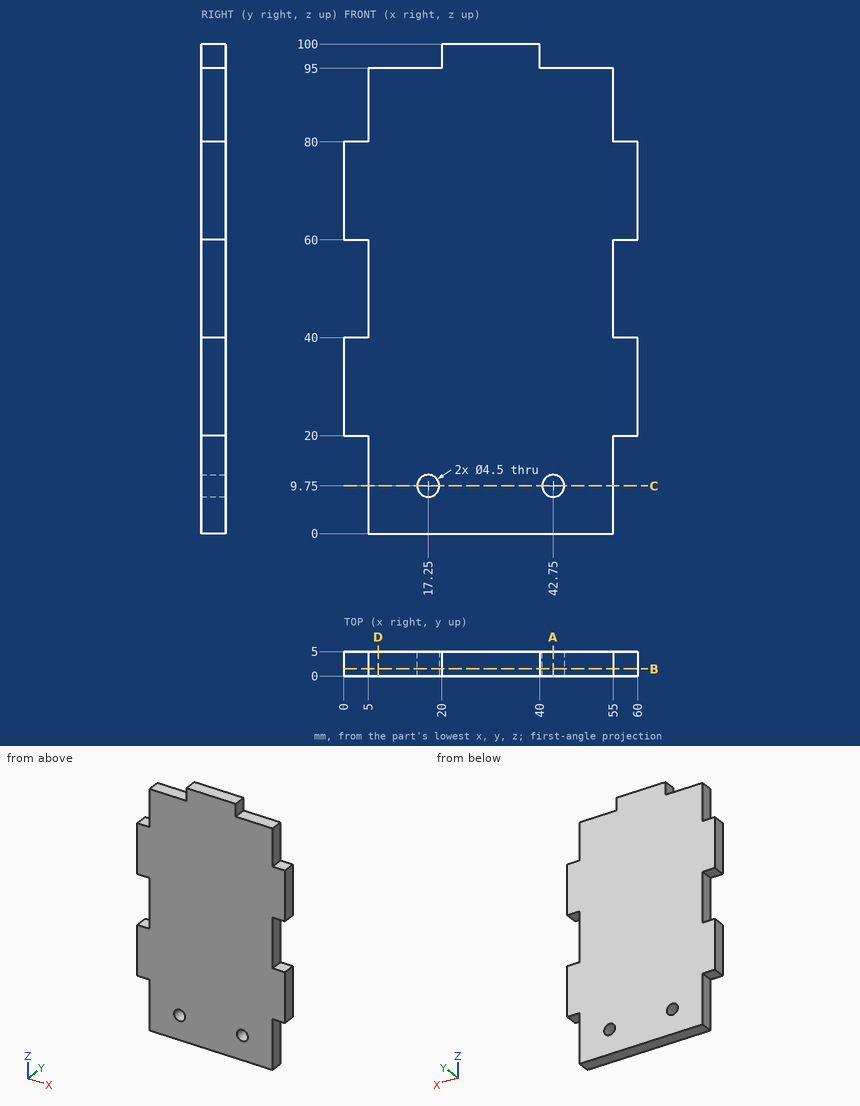
Check sheet for the drawn part. Datum: minimum x, y, z corner. Units: mm. Round coordinates to 2 decimals unless told otherwise and drop trailing zeros. Order: outer loops, then holes, each group sorted by start corner. A loop starts at its lowest first (then second) coordinate and runs counter-clockwise, first axis right, second up. Notation, with made-up numbers: M 46,28 L 72,28 A22 cw 72,34 Z; hole C 54,61.25 d1. An arc over 180 degrees is marked long. Write each question's results on one line, items separated by ' | '. Start each with the question number.
1. Cross-section at D-D on x = 7. Record the boundary of the cut face in (y, z).
2. Cross-section at B-B on y = 1.45. Record the boundary of the cut face in (x, z).
3. Material ranges on L1, parallel to Z at x = 57, y = 1.7; L2, parallel to X at y = 3.4, z = 10; L3, parallel to Z at x = 42.75, y = 2.05, recorded low to high. Write a range as from..to.
4. Cross-section at C-C on z = 9.75. Record the boundary of the cut face in (x, y).
5. Go/stop test with flat-tipped pins: P1, Ø2.5, axis at y = 3.5, z = 11.5, coming from the -X side; P2, Ø2.5, axis at x = 2.5, y = 3.5, coming from the -Z side; P3, Ø1.5, axis at y = 3.5, z = 5.5, coming from the +X side. Record where each tip stops, or that it passes through.
6. Cross-section at A-A on x = 42.75. Record the boundary of the cut face in (y, z), plus the area to 4 significant figures.
Resolved:
1) outline: M 0,0 L 5,0 L 5,95 L 0,95 Z
2) outline: M 0,20 L 5,20 L 5,0 L 55,0 L 55,20 L 60,20 L 60,40 L 55,40 L 55,60 L 60,60 L 60,80 L 55,80 L 55,95 L 40,95 L 40,100 L 20,100 L 20,95 L 5,95 L 5,80 L 0,80 L 0,60 L 5,60 L 5,40 L 0,40 Z; hole C 17.25,9.75 d4.5; hole C 42.75,9.75 d4.5
3) L1: 20..40, 60..80 | L2: 5..15.01, 19.49..40.51, 44.99..55 | L3: 0..7.5, 12..95
4) outline: M 5,0 L 15,0 L 15,5 L 5,5 Z; M 19.5,0 L 40.5,0 L 40.5,5 L 19.5,5 Z; M 45,0 L 55,0 L 55,5 L 45,5 Z
5) P1: x = 5 | P2: z = 20 | P3: x = 55
6) outline: M 0,0 L 5,0 L 5,7.5 L 0,7.5 Z; M 0,12 L 5,12 L 5,95 L 0,95 Z | area: 452.5 mm2
